The figure shows three views and two pictorial views of one solid part (mm, origin at its lowest corner). Answer the questions. A direction names the side the tool comes from. Coordinates: 2 decimals unless noted, no trailing zeros. Order: outer loops, then holes, each group sorted by start corner. A loop starts at its lowest first (then second) coordinate and runs counter-clockwise, first axis right, second up. Notation, with made-up numbers: (83, -21.5) -> (136, -21.5) arc R22 ccw to (136, 6.5) -> close; hole circle Ø6 at (32, 7.25). An arc over 180 degrees is marked (long way). Return JSON: item names as keys, results as strings.
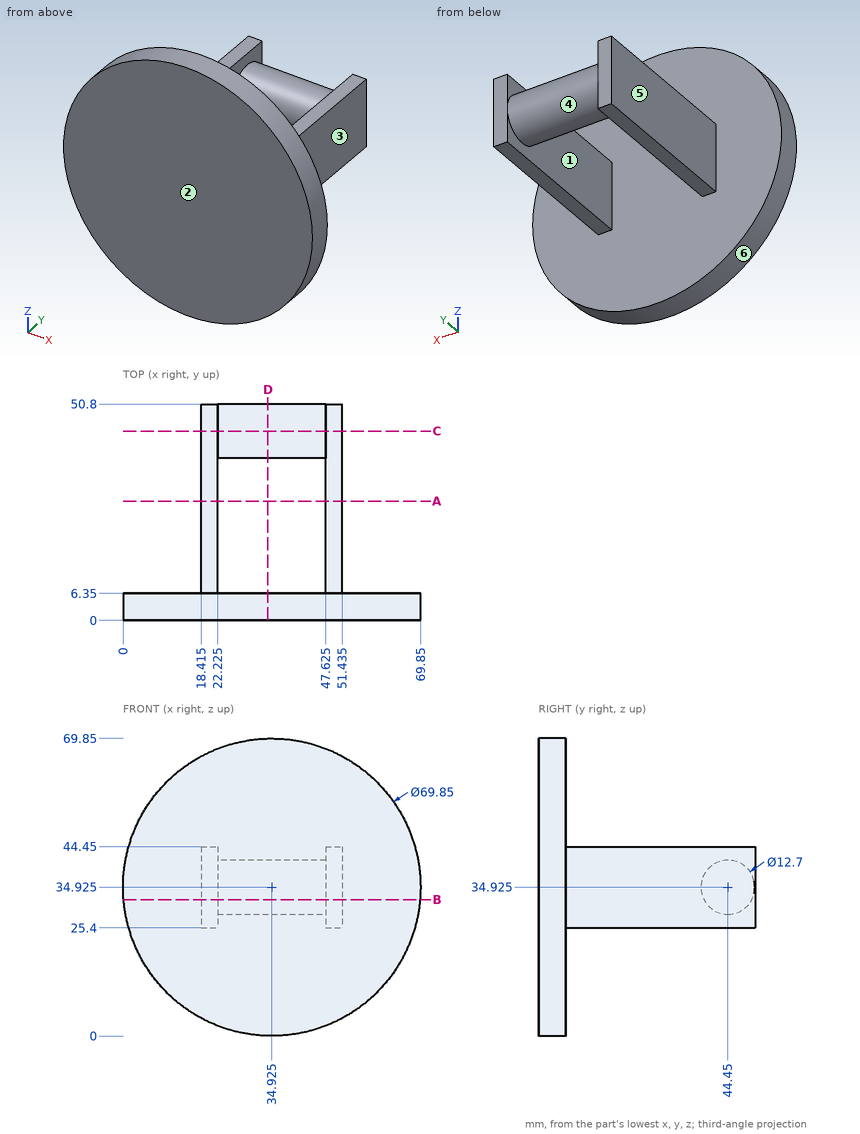
1. Determine the mould class of the marked faces 1, 2 and 3 for opening direction X: pulls with the +X half, pulls with the -X half, needs draft (parallel to the pull), parting line crosses it, or undercut.
Answer block:
{"face 1": "undercut", "face 2": "needs draft", "face 3": "pulls with the +X half"}
2. The part is cut by section C-C on y = 44.45. Give the vertices of the cut face in (x, z) (3 decimals).
Answer block:
{"outline": "(18.415, 25.4) -> (22.225, 25.4) -> (22.225, 28.575) -> (47.625, 28.575) -> (47.625, 25.4) -> (51.435, 25.4) -> (51.435, 44.45) -> (47.625, 44.45) -> (47.625, 41.275) -> (22.225, 41.275) -> (22.225, 44.45) -> (18.415, 44.45) -> close"}
3. For the marked faces 4, 5 and 6, determine the directions among +Z, -Z, +X, -X, +Y, -Y from which every point of the face is accessible in a straight line to the end or side of a thin tool.
Answer block:
{"face 4": "none", "face 5": "+Z, -Z, -X, +Y", "face 6": "+Y, -Y"}
4. The part is cut by section D-D on x = 34. Give the vertices of the cut face in (y, z) (3 decimals), and give its area (3 significant figures).
Answer block:
{"outline": "(0, 0.012) -> (6.35, 0.012) -> (6.35, 69.838) -> (0, 69.838) -> close; circle Ø12.7 at (44.45, 34.925)", "area": "570 mm2"}
5. Each of these flat-tipped pins is pushed along its axis until it touches: pin 1 Ø3 at (y, z) = (25.5, 32) entering from -X (3 decimals); pin 2 Ø2 at (x, y) = (50.5, 10.5) entering from -Z; pin 3 Ø10 at (x, z) = (61, 27.5) entering from +Y. Where does it stop, or does it pass through?
Answer block:
{"pin 1": "stops at x = 18.415", "pin 2": "stops at z = 25.4", "pin 3": "stops at y = 6.35"}
6. Consider line 1 (X direction, y = 15, z = 33) (3 decimals); line 2 (Y direction, x = 5, z = 47.5); line 3 (Z direction, x = 47.5, y = 44.5). Determine where each line is inside the solid, lowest interval first. Write a range as from..to.
Answer block:
{"line 1": "x = 18.415..22.225, 47.625..51.435", "line 2": "y = 0..6.35", "line 3": "z = 28.58..41.27"}
7. The part is cut by section B-B on z = 32. Give the vertices of the cut face in (x, y) (3 decimals), and give its area (3 significant figures).
Answer block:
{"outline": "(0.123, 0) -> (69.727, 0) -> (69.727, 6.35) -> (51.435, 6.35) -> (51.435, 50.8) -> (47.625, 50.8) -> (47.625, 50.086) -> (22.225, 50.086) -> (22.225, 50.8) -> (18.415, 50.8) -> (18.415, 6.35) -> (0.123, 6.35) -> close; hole (22.225, 6.35) -> (47.625, 6.35) -> (47.625, 38.814) -> (22.225, 38.814) -> close", "area": "1,070 mm2"}
8. The part is cut by section A-A on y = 28. Give the vertices of the cut face in (x, z) (3 decimals), and give its area (3 significant figures).
Answer block:
{"outline": "(18.415, 25.4) -> (22.225, 25.4) -> (22.225, 44.45) -> (18.415, 44.45) -> close; (47.625, 25.4) -> (51.435, 25.4) -> (51.435, 44.45) -> (47.625, 44.45) -> close", "area": "145 mm2"}
